Work out the finished part from the listing and answer in its coordinate system (mm). Give positions to 0.01 mm unless a question says otherwise; leave off trailing zeros. Loops run counter-clockwise (first coordinate to the right, second up) from the corner with the lowest first, then second, coordinate; pieces in that order, holes last.
```python
from build123d import *

# Parameters (mm, degrees)
SKETCH_2_W = 450
SKETCH_2_H = 2


with BuildPart() as part:
    # 扫描1: sweep along a path in 草图1
    with BuildLine(Plane.XY) as sweep_1_path:
        Line((0, 0), (0, 700))
        ThreePointArc((0, 700), (1194.974746831, 1194.974746831), (700, 0))
        Line((700, 0), (0, 0))
    # 草图2 → 扫描1 (sweep)
    with BuildSketch(Plane(origin=(0, 0, 0), x_dir=(1, 0, 0), z_dir=(0, 1, 0))):
        Rectangle(SKETCH_2_W, SKETCH_2_H)
    sweep(path=sweep_1_path.line, transition=Transition.RIGHT)


solid = part.part
```
Q1. Determine the mould class of faces 1 (the face through (1332.146, 1375.29, 0.014)), 2 (the face through (919, 1124, -1)), 3 (the face through (1024.616, 1046.77, -0.014)) for opening direction Y: +Y half, -Y half, draft (parallel to the pull), parting line (faces both ways), or undercut.
Q2. Section D-D on x = 1269 is taken. Give the vertices of the cut face in (y, z), plus the area to 3 significant figures.
Q3. Given pin 1 (1 mm diameter, centred on y = 1354, z = 0, fed in from +X); pin 2 (1 mm diameter, centred on x = 537.5, z = -0.5, fed in from +Y); pin 3 (0.6 mm diameter, centred on y = 501, z = -0.5, fed in from +X), each flat-ended and moving along its own axis, determine where each tip first touches the part or whether it passes through.
Q4. Section C-C on x = 813.5 is taken. Give the vertices of the cut face in (y, z).
Q5. Section B-B on y = 340 is taken. Give the vertices of the cut face in (x, z).
Q6. Consider line 1 along X through (y, z) = (700, -0.3); line 2 along Y through (x, z) = (720, 0); line 3 along X through (y, z) = (978, -0.15). Determine where each line is inside the solid, lowest interval first.
Q7. Section A-A on z = 0.25 is taken. Give the vertices of the cut face in (x, y).
Check result:
1. face 1: parting line
1. face 2: draft
1. face 3: undercut
2. outline: (-29.29, -1) - (1429.29, -1) - (1429.29, 1) - (-29.29, 1) - close
2. area: 2,920 mm2
3. pin 1: stops at x = 1354.65
3. pin 2: stops at y = 1610.7
3. pin 3: stops at x = 1603.41
4. outline: (-218.01, -1) - (238.76, -1) - (238.76, 1) - (-218.01, 1) - close; (1161.24, -1) - (1618.01, -1) - (1618.01, 1) - (1161.24, 1) - close
5. outline: (-225, -1) - (225, -1) - (225, 1) - (-225, 1) - close; (1009.88, -1) - (1552.07, -1) - (1552.07, 1) - (1009.88, 1) - close
6. line 1: x = -225 to 225, 1175 to 1625
6. line 2: y = -224.78 to 225.42, 1174.58 to 1624.78
6. line 3: x = -182.24 to 314.85, 1085.15 to 1582.24
7. outline: (-225, -225) - (700, -225) arc R925 ccw (long way) to (-225, 700) - close; hole (225, 225) - (700, 225) arc R475 ccw (long way) to (225, 700) - close
